```python
from build123d import *

# Parameters (mm, degrees)
SKETCH1_R           = 4.7879
SKETCH1_R_2         = 3.2004
BOSS_EXTRUDE1_DEPTH = 4.7498
SKETCH2_R           = 6.35
SKETCH2_R_2         = 3.2004
BOSS_EXTRUDE2_DEPTH = 1.6002
CHAMFER1_SIZE       = 0.254


with BuildPart() as part:
    # Sketch1 → Boss-Extrude1 (new body)
    with BuildSketch(Plane(origin=(0, 0, 0), x_dir=(0, 0, -1), z_dir=(1, 0, 0))):
        Circle(SKETCH1_R)
        Circle(SKETCH1_R_2, mode=Mode.SUBTRACT)
    extrude(amount=BOSS_EXTRUDE1_DEPTH)

    # Sketch2 → Boss-Extrude2 (add)
    with BuildSketch(Plane.ZY):
        Circle(SKETCH2_R)
        Circle(SKETCH2_R_2, mode=Mode.SUBTRACT)
    extrude(amount=BOSS_EXTRUDE2_DEPTH)

    # Chamfer1
    chamfer1_edges = [part.edges().sort_by_distance(p)[0] for p in [
        (-1.6002, 0, -3.2004),
        (4.7498, 0, 3.2004),
    ]]
    chamfer(chamfer1_edges, length=CHAMFER1_SIZE)


solid = part.part
```
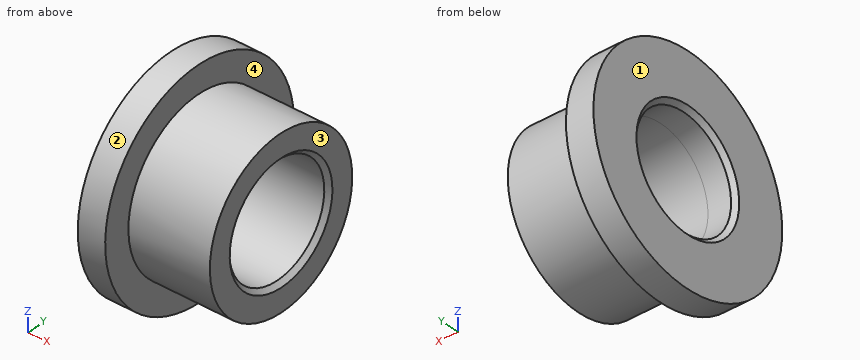
Read the model definition and answer for the solid it produces. Units are mm, in the model's axes. Face numbers are marked on the shaded views. A direction names the side the tool comes from. Give positions to 0.01 mm unless a question says otherwise; leave off trailing zeros. Order: outer loops, then holes, each group sorted by start corner. A loop starts at its lowest first (then second) coordinate and runs counter-clockwise, first axis right, second up.
(1) For the marked faces 3 and 4, determine the directions among +Z, -Z, +X, -X, +Y, -Y from which every point of the face is accessible in a straight line to the end or side of a thin tool.
(2) Given pin 1 (3 mm diameter, centred on x = 0, y = -4.5, fed in from +Z); pin 2 (1 mm diameter, centred on x = -1, y = -1, fed in from -Z); pin 3 (7.5 mm diameter, centred on y = 0, z = 0, fed in from +X), each flat-ended and moving along its own axis, determine where each tip first touches the part or whether it passes through.
(3) Find section D-D (y = 4). Give the vertices of the cut face in (x, z).
(4) Find section C-C (x = 1.25). Give the vertices of the cut face in (y, z).
(5) For a pull along Z with two mould halves and no side action, classify the marked faces 1 and 2 as released by +Z, released by -Z, zero draft, split by the parting line, or undercut.
(6) Find section A-A (y = 0). Give the vertices of the cut face in (x, z), plus the area to 3 significant figures.
(7) Straight lines are drawn through the part: L1, parallel to Y at x = 3.5, z = 0; L2, parallel to Y at x = -0.95, z = 0; L3, parallel to X at y = -5.25, z = 3. For each, find the intervals that lie inside material, in ascending order.
Result sheet:
1. face 3: +Z, -Z, +X, +Y, -Y
1. face 4: +X
2. pin 1: stops at z = 5.6
2. pin 2: stops at z = -6.33
2. pin 3: stops at x = 4.75
3. outline: (-1.6, -4.93) - (0, -4.93) - (0, -2.63) - (4.75, -2.63) - (4.75, 2.63) - (0, 2.63) - (0, 4.93) - (-1.6, 4.93) - close
4. outline: circle Ø9.58 at (0, 0); hole circle Ø6.4 at (0, 0)
5. face 1: zero draft
5. face 2: split by the parting line
6. outline: (-1.6, -6.35) - (0, -6.35) - (0, -4.79) - (4.75, -4.79) - (4.75, -3.45) - (4.5, -3.2) - (-1.35, -3.2) - (-1.6, -3.45) - close; (-1.6, 3.45) - (-1.35, 3.2) - (4.5, 3.2) - (4.75, 3.45) - (4.75, 4.79) - (0, 4.79) - (0, 6.35) - (-1.6, 6.35) - close
6. area: 25.0 mm2
7. L1: y = -4.79 to -3.2, 3.2 to 4.79
7. L2: y = -6.35 to -3.2, 3.2 to 6.35
7. L3: x = -1.6 to 0
